from build123d import *

# Parameters (mm, degrees)
SKETCH1_W               = 120
SKETCH1_H               = 80
BOSS_EXTRUDE1_DEPTH     = 25
SKETCH2_W               = 116.6
SKETCH2_H               = 76.6
CUT_EXTRUDE1_DEPTH      = 24
SKETCH4_R               = 2.25
BOSS_EXTRUDE3_DEPTH     = 3
SKETCH6_W               = 5.06
SKETCH6_H               = 2
BOSS_EXTRUDE4_DEPTH     = 12
SKETCH7_R               = 1.75
BOSS_EXTRUDE5_DEPTH     = 10
SKETCH8_R               = 5
BOSS_EXTRUDE6_DEPTH     = 5
SKETCH9_R               = 4
CUT_EXTRUDE2_DEPTH      = 2.5
MIRROR2_COPY_1_SKETCH_R = 5
MIRROR2_COPY_1_DEPTH    = 5
MIRROR2_COPY_2_SKETCH_R = 4
MIRROR2_COPY_2_DEPTH    = 2.5
FILLET1_R               = 3
SKETCH10_R              = 2.25
CUT_EXTRUDE3_DEPTH      = 2
CUT_EXTRUDE4_REACH      = 157.234
SKETCH11_W              = 12
SKETCH11_H              = 4.5
CUT_EXTRUDE5_DEPTH      = 156.233896105
CUT_EXTRUDE5_DEPTH_BACK = 156.233896105
CUT_EXTRUDE6_START      = -1.7
CUT_EXTRUDE6_DEPTH      = 157.933896105
MIRROR3_START           = 3
MIRROR3_OUTLINE_W       = 1.7
MIRROR3_OUTLINE_H       = 6.070107007
MIRROR3_OUTLINE_H_2     = 6
MIRROR3_DEPTH           = 6


# Read off the part's stored shape, not the designer's step: Mirror3
with BuildPart() as part:
    # Sketch1 → Boss-Extrude1 (new body)
    with BuildSketch(Plane.XY):
        with Locations((60, 40)):
            Rectangle(SKETCH1_W, SKETCH1_H)
    extrude(amount=BOSS_EXTRUDE1_DEPTH)

    # Sketch2 → Cut-Extrude1 (cut)
    with BuildSketch(Plane.XY.offset(25)):
        with Locations((60, 40)):
            Rectangle(SKETCH2_W, SKETCH2_H)
    extrude(amount=-CUT_EXTRUDE1_DEPTH, mode=Mode.SUBTRACT)

    # Sketch4 → Boss-Extrude3 (add)
    # profile 1 of 2: a face of its own
    with BuildSketch(Plane(origin=(0, 0, 0), x_dir=(-1, 0, 0), z_dir=(0, 0, -1))):
        with BuildLine():
            Line((-68, 80), (-68, 87.25))
            ThreePointArc((-68, 87.25), (-60, 95.25), (-52, 87.25))
            Line((-52, 87.25), (-52, 80))
            Line((-52, 80), (-68, 80))
        make_face()
        with Locations((-60, 87.25)):
            Circle(SKETCH4_R, mode=Mode.SUBTRACT)
    # profile 2 of 2: a face of its own
    with BuildSketch(Plane(origin=(0, 0, 0), x_dir=(-1, 0, 0), z_dir=(0, 0, -1))):
        with BuildLine():
            Line((-68, 0), (-68, -7.25))
            ThreePointArc((-68, -7.25), (-60, -15.25), (-52, -7.25))
            Line((-52, -7.25), (-52, 0))
            Line((-52, 0), (-68, 0))
        make_face()
        with Locations(Location((-60, -7.25, 0), (0, 0, 180))):
            Circle(SKETCH4_R, mode=Mode.SUBTRACT)
    extrude(amount=-BOSS_EXTRUDE3_DEPTH)

    # Sketch6 → Boss-Extrude4 (add)
    with BuildSketch(Plane.XY):
        Polygon((90.44, 78.3), (92.44, 78.3), (92.44, 38.89), (98.04, 38.89), (98.04, 36.89), (90.44, 36.89), align=None)
        with Locations((115.77, 37.89)):
            Rectangle(SKETCH6_W, SKETCH6_H)
    extrude(amount=BOSS_EXTRUDE4_DEPTH)

    # Sketch7 → Boss-Extrude5 (add)
    with BuildSketch(Plane.XY.offset(1)):
        with Locations((44.85, 69)):
            Circle(SKETCH7_R)
        with Locations((44.85, 11)):
            Circle(SKETCH7_R)
        with Locations((76.85, 69)):
            Circle(SKETCH7_R)
        with Locations((76.85, 11)):
            Circle(SKETCH7_R)
    extrude(amount=BOSS_EXTRUDE5_DEPTH)

    # Sketch8 → Boss-Extrude6 (add)
    with BuildSketch(Plane.XY.offset(25)):
        with Locations((5, 75)):
            Circle(SKETCH8_R)
    boss_extrude6 = extrude(amount=-BOSS_EXTRUDE6_DEPTH)

    # Sketch9 → Cut-Extrude2 (cut)
    with BuildSketch(Plane.XY.offset(25)):
        with Locations((5, 75)):
            Circle(SKETCH9_R)
    cut_extrude2 = extrude(amount=-CUT_EXTRUDE2_DEPTH, mode=Mode.SUBTRACT)

    # Mirror1: Boss-Extrude6, Cut-Extrude2 across plane
    add(boss_extrude6.mirror(Plane.ZY.offset(-60)))
    add(cut_extrude2.mirror(Plane.ZY.offset(-60)), mode=Mode.SUBTRACT)

    # Mirror2: Boss-Extrude6, Cut-Extrude2 across plane
    add(boss_extrude6.mirror(Plane.ZX.offset(40)))
    add(cut_extrude2.mirror(Plane.ZX.offset(40)), mode=Mode.SUBTRACT)

    # Mirror2 copy 1 sketch → Mirror2 copy 1 (add)
    with BuildSketch(Plane(origin=(120, 80, 25), x_dir=(-1, 0, 0), z_dir=(0, 0, 1))):
        with Locations((5, 75)):
            Circle(MIRROR2_COPY_1_SKETCH_R)
    extrude(amount=-MIRROR2_COPY_1_DEPTH)

    # Mirror2 copy 2 sketch → Mirror2 copy 2 (cut)
    with BuildSketch(Plane(origin=(120, 80, 25), x_dir=(-1, 0, 0), z_dir=(0, 0, 1))):
        with Locations((5, 75)):
            Circle(MIRROR2_COPY_2_SKETCH_R)
    extrude(amount=-MIRROR2_COPY_2_DEPTH, mode=Mode.SUBTRACT)

    # Fillet1
    fillet1_edges = [part.edges().sort_by_distance(p)[0] for p in [
        (0, 80, 12.5),
        (120, 80, 12.5),
        (120, 0, 12.5),
        (0, 0, 12.5),
    ]]
    fillet(fillet1_edges, radius=FILLET1_R)

    # Sketch10 → Cut-Extrude3 (cut)
    with BuildSketch(Plane(origin=(0, 0, 0), x_dir=(-1, 0, 0), z_dir=(0, 0, -1))):
        with Locations((-28.5, 71.5)):
            Circle(SKETCH10_R)
        with Locations((-12.75, 55.75)):
            Circle(SKETCH10_R)
        with Locations((-28.5, 55.75)):
            Circle(SKETCH10_R)
        with Locations((-12.75, 40)):
            Circle(SKETCH10_R)
        with Locations((-28.5, 40)):
            Circle(SKETCH10_R)
        with Locations((-44.25, 40)):
            Circle(SKETCH10_R)
        with Locations((-12.75, 24.25)):
            Circle(SKETCH10_R)
        with Locations((-28.5, 24.25)):
            Circle(SKETCH10_R)
        with Locations((-44.25, 24.25)):
            Circle(SKETCH10_R)
        with Locations((-12.75, 8.5)):
            Circle(SKETCH10_R)
        with BuildLine():
            ThreePointArc((-57.75, 24.25), (-58.409009742, 25.840990258), (-60, 26.5))
            Line((-60, 26.5), (-60, 22))
            ThreePointArc((-60, 22), (-58.409009742, 22.659009742), (-57.75, 24.25))
        make_face()
        with BuildLine():
            Line((-60, 22), (-60, 26.5))
            ThreePointArc((-60, 26.5), (-62.25, 24.25), (-60, 22))
        make_face()
        with BuildLine():
            ThreePointArc((-57.75, 8.5), (-58.409009742, 10.090990258), (-60, 10.75))
            Line((-60, 10.75), (-60, 6.25))
            ThreePointArc((-60, 6.25), (-58.409009742, 6.909009742), (-57.75, 8.5))
        make_face()
        with BuildLine():
            Line((-60, 6.25), (-60, 10.75))
            ThreePointArc((-60, 10.75), (-62.25, 8.5), (-60, 6.25))
        make_face()
        with BuildLine():
            ThreePointArc((-57.75, 40), (-58.409009742, 41.590990258), (-60, 42.25))
            Line((-60, 42.25), (-60, 37.75))
            ThreePointArc((-60, 37.75), (-58.409009742, 38.409009742), (-57.75, 40))
        make_face()
        with BuildLine():
            Line((-60, 37.75), (-60, 42.25))
            ThreePointArc((-60, 42.25), (-62.25, 40), (-60, 37.75))
        make_face()
        with BuildLine():
            ThreePointArc((-57.75, 55.75), (-58.409009742, 57.340990258), (-60, 58))
            Line((-60, 58), (-60, 53.5))
            ThreePointArc((-60, 53.5), (-58.409009742, 54.159009742), (-57.75, 55.75))
        make_face()
        with BuildLine():
            Line((-60, 53.5), (-60, 58))
            ThreePointArc((-60, 58), (-62.25, 55.75), (-60, 53.5))
        make_face()
        with BuildLine():
            ThreePointArc((-57.75, 71.5), (-58.409009742, 73.090990258), (-60, 73.75))
            Line((-60, 73.75), (-60, 69.25))
            ThreePointArc((-60, 69.25), (-58.409009742, 69.909009742), (-57.75, 71.5))
        make_face()
        with BuildLine():
            Line((-60, 69.25), (-60, 73.75))
            ThreePointArc((-60, 73.75), (-62.25, 71.5), (-60, 69.25))
        make_face()
        with Locations((-75.75, 24.25)):
            Circle(SKETCH10_R)
        with Locations((-75.75, 55.75)):
            Circle(SKETCH10_R)
        with Locations((-75.75, 40)):
            Circle(SKETCH10_R)
        with Locations((-91.5, 24.25)):
            Circle(SKETCH10_R)
        with Locations((-107.25, 24.25)):
            Circle(SKETCH10_R)
        with Locations((-107.25, 8.5)):
            Circle(SKETCH10_R)
        with Locations((-107.25, 55.75)):
            Circle(SKETCH10_R)
        with Locations((-107.25, 40)):
            Circle(SKETCH10_R)
        with Locations((-12.75, 71.5)):
            Circle(SKETCH10_R)
        with Locations((-44.25, 55.75)):
            Circle(SKETCH10_R)
        with Locations((-28.5, 8.5)):
            Circle(SKETCH10_R)
        with Locations((-60, 8.5)):
            Circle(SKETCH10_R)
        with Locations((-91.5, 8.5)):
            Circle(SKETCH10_R)
        with Locations((-107.25, 71.5)):
            Circle(SKETCH10_R)
    extrude(amount=-CUT_EXTRUDE3_DEPTH, mode=Mode.SUBTRACT)

    # Sketch11 → Cut-Extrude4 (cut, up to next)
    with BuildSketch(Plane(origin=(0, 80, 0), x_dir=(1, 0, 0), z_dir=(0, 1, 0)), mode=Mode.PRIVATE) as cut_extrude4_sk1:
        with Locations((105, -3.25)):
            Rectangle(SKETCH11_W, SKETCH11_H)
    cut_extrude4_tool1 = extrude(cut_extrude4_sk1.sketch, amount=-CUT_EXTRUDE4_REACH, mode=Mode.PRIVATE) & part.part
    add(cut_extrude4_tool1.solids().sort_by_distance((105, 80, 3.25))[0], mode=Mode.SUBTRACT)

    # Sketch12 → Cut-Extrude5 (cut, two sides: drawn at the far end of the back side and taken through both)
    with BuildSketch(Plane.XZ.offset(-CUT_EXTRUDE5_DEPTH_BACK)):
        Polygon((60, 3), (54, 3), (54, 9), (60, 9), (66, 9), (66, 3), align=None)
    extrude(amount=CUT_EXTRUDE5_DEPTH + CUT_EXTRUDE5_DEPTH_BACK, mode=Mode.SUBTRACT)

    # Sketch13 → Cut-Extrude6 (cut)
    with BuildSketch(Plane.ZY.offset(CUT_EXTRUDE6_START)):
        Polygon((3, 40), (3, 43), (9, 43), (9, 40), (9, 37), (3, 37), align=None)
        Polygon((3, 65), (3, 69.070107007), (9, 69.070107007), (9, 66), (9, 63), (3, 63), align=None)
        Polygon((3, 17), (3, 11), (9, 11), (9, 15.086809652), (9, 17), align=None)
    extrude(amount=CUT_EXTRUDE6_DEPTH, mode=Mode.SUBTRACT)

    # Mirror3 outline → Mirror3 (cut)
    with BuildSketch(Plane.XY.offset(MIRROR3_START)):
        with Locations((119.15, 66.035053504)):
            Rectangle(MIRROR3_OUTLINE_W, MIRROR3_OUTLINE_H)
        with Locations((119.15, 14)):
            Rectangle(MIRROR3_OUTLINE_W, MIRROR3_OUTLINE_H_2)
    extrude(amount=MIRROR3_DEPTH, mode=Mode.SUBTRACT)


solid = part.part
For this review, take the finished solid that the model builds, in its own axes (mm). A direction names the side the tool comes from. Coordinates: 2 decimals unless noted, no trailing zeros. Loops run counter-clockwise (first coordinate to the right, second up) from the corner with the lowest first, then second, coordinate; pieces in that order, holes last. Notation, with made-up numbers: (-27.75, -32.75) - (-10.75, -32.75) arc R20 cw to (-10.75, -16.75) - close; hole circle Ø7 at (85.5, 15). An arc over 180 degrees is marked (long way). Use a Markdown table: item, result. Add a question column.
Item 1: We need section A-A (x = 107.25). Give the number of separate pieces and of enclosed holes in the cut face, and give its area (3 significant figures).
Item 2: We need section C-C (x = 28.5). Give the boundary of the cut face in (y, z).
Item 3: We need section D-D (y = 60.5). Give the boundary of the cut face in (x, z).
Item 4: Insertion check: pin 1 Ø6 at (x, z) = (94.5, 7) entering from +Y; pin 2 Ø2.5 at (x, z) = (116, 7) entering from -Y; pin 3 Ø5 at (x, y) = (12.75, 8.5) entering from +Z. Each pin has a flat end and moves straight along its axis. Give the tip position at first contact, or say it passes through.
Item 5: Mouldability with a two-part tool opening along X and no side actions: class faces 4 (the face through (114, 6, 20)), 5 (the face through (59, 0, 12)), 6 (the face through (60.176, -15.248, 1.479)) as pulls with the +X half, pulls with the -X half, needs draft (parallel to the pull), parting line crosses it, or undercut.
Item 6: For line 1 (Y direction, x = 93.5, z = 1.75); line 2 (X direction, y = 44, z = 1.5); line 3 (Y direction, x = 107.25, z = 0.4), list the stretches that pass through material, from the lowest coordinate up.
Item 7: We need section B-B (z = 14.25). Give the boundary of the cut face in (x, y), and give its area (3 significant figures).
Item 8: Tool access review of faces 1 (the face through (6, 74, 20)), 2 (the face through (46.519, 11.526, 5.93)), 3 (the face through (45.91, 57.27, 0.49)): name each direction out of +Z, -Z, +X, -X, +Y, -Y from which nothing blocks a thin tool from reaching the whole face with its end or side.
Results list:
| question | item | result |
|---|---|---|
| 1 | separate pieces | 7 |
| 1 | enclosed holes | 0 |
| 1 | area | 131 mm^2 |
| 2 | outline | (0, 0) - (6.25, 0) - (6.25, 1) - (1.7, 1) - (1.7, 25) - (0, 25) - close; (10.75, 0) - (22, 0) - (22, 1) - (10.75, 1) - close; (26.5, 0) - (37.75, 0) - (37.75, 1) - (26.5, 1) - close; (42.25, 0) - (53.5, 0) - (53.5, 1) - (42.25, 1) - close; (58, 0) - (69.25, 0) - (69.25, 1) - (58, 1) - close; (73.75, 0) - (80, 0) - (80, 25) - (78.3, 25) - (78.3, 1) - (73.75, 1) - close |
| 3 | outline | (0, 0) - (120, 0) - (120, 25) - (118.3, 25) - (118.3, 1) - (92.44, 1) - (92.44, 12) - (90.44, 12) - (90.44, 1) - (1.7, 1) - (1.7, 25) - (0, 25) - close |
| 4 | pin 1 | stops at y = 80 |
| 4 | pin 2 | stops at y = 0 |
| 4 | pin 3 | stops at z = 1 |
| 5 | face 4 | undercut |
| 5 | face 5 | needs draft |
| 5 | face 6 | parting line crosses it |
| 6 | line 1 | y = 0 to 1.7, 36.89 to 38.89, 78.3 to 80 |
| 6 | line 2 | x = 0 to 1.7, 90.44 to 92.44, 118.3 to 120 |
| 6 | line 3 | y = 0 to 6.25, 10.75 to 22, 26.5 to 37.75, 42.25 to 53.5, 58 to 69.25, 73.75 to 80 |
| 7 | outline | (0, 3) arc R3 ccw to (3, 0) - (117, 0) arc R3 ccw to (120, 3) - (120, 77) arc R3 ccw to (117, 80) - (3, 80) arc R3 ccw to (0, 77) - close; hole (1.7, 1.7) - (118.3, 1.7) - (118.3, 78.3) - (1.7, 78.3) - close |
| 7 | area | 661 mm^2 |
| 8 | face 1 | none |
| 8 | face 2 | +Z |
| 8 | face 3 | +Z, -Z |
